```python
from build123d import *

# Parameters (mm, degrees)
PAD002_DEPTH    = 5.1
PAD003_DEPTH    = 5.1
PAD001_DEPTH    = 5.1
SKETCH_W        = 70
SKETCH_H        = 55
PAD_DEPTH       = 10
SKETCH001_R     = 11.05
POCKET_DEPTH    = 7
SKETCH002_R     = 5
POCKET001_DEPTH = 3.001
SKETCH003_W     = 12
SKETCH003_H     = 8.1
SKETCH003_W_2   = 8
SKETCH003_H_2   = 12
POCKET002_DEPTH = 10.001
SKETCH004_R     = 2.1
POCKET003_DEPTH = 10
SKETCH005_R     = 2.1
POCKET004_DEPTH = 10
SKETCH006_R     = 2.1
POCKET005_DEPTH = 10
SKETCH010_W     = 70
SKETCH010_H     = 13
POCKET006_DEPTH = 10.001
SKETCH011_R     = 9
SKETCH011_R_2   = 6
SKETCH011_R_3   = 7
SKETCH011_R_4   = 2.6
PAD004_DEPTH    = 0.3
SKETCH012_R     = 5
PAD005_DEPTH    = 0.3


with BuildPart() as pad002:
    # Sketch008 → Pad002 (new body)
    with BuildSketch(Plane.YZ.offset(24)):
        Polygon((7.570319, 5), (5.53516, 8.525), (1.46484, 8.525), (-0.570319, 5), (-0.570319, 0), (7.570319, 0), align=None)
    extrude(amount=-PAD002_DEPTH)


with BuildPart() as pad003:
    # Sketch009 → Pad003 (new body)
    with BuildSketch(Plane.XZ.offset(16.5)):
        Polygon((-24.929681, 5), (-26.96484, 8.525), (-31.03516, 8.525), (-33.070319, 5), (-33.070319, 0), (-24.929681, 0), align=None)
        Polygon((33.070319, 5), (31.03516, 8.525), (26.96484, 8.525), (24.929681, 5), (24.929681, 0), (33.070319, 0), align=None)
    extrude(amount=-PAD003_DEPTH)


with BuildPart() as pad001:
    # Sketch007 → Pad001 (new body)
    with BuildSketch(Plane.YZ.offset(-24)):
        Polygon((7.570319, 5), (5.53516, 8.525), (1.46484, 8.525), (-0.570319, 5), (-0.570319, 0), (7.570319, 0), align=None)
    extrude(amount=PAD001_DEPTH)


with BuildPart() as obj1:
    # Sketch → Pad (new body)
    with BuildSketch(Plane.XY):
        Rectangle(SKETCH_W, SKETCH_H)
    extrude(amount=PAD_DEPTH)

    # Sketch001 → Pocket (cut)
    with BuildSketch(Plane(origin=(0, 0, 0), x_dir=(1, 0, 0), z_dir=(0, 0, -1))):
        with Locations((0, 13.45)):
            Circle(SKETCH001_R)
    extrude(amount=-POCKET_DEPTH, mode=Mode.SUBTRACT)

    # Sketch002 → Pocket001 (cut, through all)
    with BuildSketch(Plane(origin=(0, 0, 7), x_dir=(1, 0, 0), z_dir=(0, 0, -1))):
        with Locations((0, 13.45)):
            Circle(SKETCH002_R)
    extrude(amount=-POCKET001_DEPTH, mode=Mode.SUBTRACT)

    # Sketch003 → Pocket002 (cut, through all)
    with BuildSketch(Plane.XY.offset(10)):
        with Locations((-29, -23.45)):
            Rectangle(SKETCH003_W, SKETCH003_H)
        with Locations((29, -23.45)):
            Rectangle(SKETCH003_W, SKETCH003_H)
        with Locations((-31, 3.5)):
            Rectangle(SKETCH003_W_2, SKETCH003_H_2)
        with Locations((31, 3.5)):
            Rectangle(SKETCH003_W_2, SKETCH003_H_2)
    extrude(amount=-POCKET002_DEPTH, mode=Mode.SUBTRACT)

    # Sketch004 → Pocket003 (cut)
    with BuildSketch(Plane(origin=(-27, 0, 0), x_dir=(0, -1, 0), z_dir=(-1, 0, 0))):
        with Locations((-3.5, 5)):
            Circle(SKETCH004_R)
    extrude(amount=-POCKET003_DEPTH, mode=Mode.SUBTRACT)

    # Sketch005 → Pocket004 (cut)
    with BuildSketch(Plane.YZ.offset(27)):
        with Locations((3.5, 5)):
            Circle(SKETCH005_R)
    extrude(amount=-POCKET004_DEPTH, mode=Mode.SUBTRACT)

    # Sketch006 → Pocket005 (cut)
    with BuildSketch(Plane.XZ.offset(19.4)):
        with Locations((-29, 5)):
            Circle(SKETCH006_R)
        with Locations((29, 5)):
            Circle(SKETCH006_R)
    extrude(amount=-POCKET005_DEPTH, mode=Mode.SUBTRACT)

    # Cut: cut Pad001
    add(pad001.part, mode=Mode.SUBTRACT)

    # Cut001: cut Pad003
    add(pad003.part, mode=Mode.SUBTRACT)

    # Cut002: cut Pad002
    add(pad002.part, mode=Mode.SUBTRACT)

    # Sketch010 → Pocket006 (cut, through all)
    with BuildSketch(Plane.XY.offset(10)):
        with Locations((0, 21)):
            Rectangle(SKETCH010_W, SKETCH010_H)
    extrude(amount=-POCKET006_DEPTH, mode=Mode.SUBTRACT)

    # Sketch011 → Pad004 (new body)
    with BuildSketch(Plane(origin=(0, 0, 0), x_dir=(1, 0, 0), z_dir=(0, 0, -1))):
        with Locations((-35, -14.5)):
            Circle(SKETCH011_R)
        with Locations((-35, 2.5)):
            Circle(SKETCH011_R_2)
        with Locations((-23, 27.5)):
            Circle(SKETCH011_R_3)
        with Locations((-35, 19.4)):
            Circle(SKETCH011_R_4)
        with Locations((35, 19.4)):
            Circle(SKETCH011_R_4)
        with Locations((23, 27.5)):
            Circle(SKETCH011_R_3)
        with Locations((35, 2.5)):
            Circle(SKETCH011_R_2)
        with Locations((35, -14.5)):
            Circle(SKETCH011_R)
    extrude(amount=-PAD004_DEPTH)

    # Sketch012 → Pad005 (new body)
    with BuildSketch(Plane(origin=(0, 0, 7), x_dir=(1, 0, 0), z_dir=(0, 0, -1))):
        with Locations((0, 13.45)):
            Circle(SKETCH012_R)
    extrude(amount=-PAD005_DEPTH)


solid = obj1.part
```
Can you work these out from the model? Positions are in its coordinate system, mm. A direction names the side the tool comes from. Coordinates: 2 decimals unless noted, no trailing zeros. Loops run counter-clockwise (first coordinate to the right, second up) from the corner with the lowest first, then second, coordinate; pieces in that order, holes last.
1) I need wall thicknesses on probe 1 along Y at (x, z) = (28.5, 2); probe 2 along Y at (x, z) = (18, 5.25); probe 3 along Z at (x, y) = (29, -18.3). Which ranges of each line are inside material? Lowest first, please.
2) Imagine slicing it at B-B on y = -30. List the corners of the cut face in (x, z) for me, plus the area to 3 significant figures.
3) Which directions (+Z, -Z, +X, -X, +Y, -Y) give clear straight access to the entire face, cutting with the end or side of a thin tool? Please do faces 3 (the cylindrical face through (-31.1, -17.97, 5.09)), 4 (the cylindrical face through (-25.521, 3.773, 7.082)), 5 (the flat face through (21, 7.57, 2)), 6 (the cylindrical face through (-0.7, -18.4, 8.6)).
4) Imagine slicing it at A-A on x = 0. List the corners of the cut face in (y, z) for me, plus the area to 3 significant figures.
5) Thinking about a two-plate mould opening in X: for faces 1 (the cylindrical face through (-17.963, 3.773, 7.082)), 2 (the flat face through (-33.07, -14, 3)), which applies, pulls with the +X half, pulls with the -X half, needs draft (parallel to the pull), parting line crosses it, or undercut?
6) Imagine slicing it at D-D on x = 9. List the corners of the cut face in (y, z) for me.
7) For pin 1 (5.5 mm diameter, centred on x = 22.5, z = 3, fed in from +Y); pin 2 (2 mm diameter, centred on x = -28, y = -22, fed in from +Z); pin 3 (1.5 mm diameter, centred on y = -14.5, z = 2, fed in from +X), each with a flat end and sliding along its axis, tell me the tip position at first contact or that it passes through.
8) Imagine slicing it at C-C on y = -7.5. List the corners of the cut face in (x, z) for me.
Completed:
1. probe 1: y = -19.4 to -16.5, -11.4 to -2.5, 9.5 to 14.5
1. probe 2: y = -27.5 to 1.41, 5.59 to 14.5
1. probe 3: z = 0 to 2.9, 7.1 to 10
2. outline: (-29.54, 0) - (-16.46, 0) - (-16.46, 0.3) - (-29.54, 0.3) - close; (16.46, 0) - (29.54, 0) - (29.54, 0.3) - (16.46, 0.3) - close
2. area: 7.85 mm2
3. face 3: -Y
3. face 4: -X
3. face 5: -Z
3. face 6: +Z
4. outline: (-27.5, 0) - (-24.5, 0) - (-24.5, 7) - (-2.4, 7) - (-2.4, 0) - (14.5, 0) - (14.5, 10) - (-8.45, 10) - (-8.45, 7.3) - (-18.45, 7.3) - (-18.45, 10) - (-27.5, 10) - close
4. area: 238 mm2
5. face 1: needs draft
5. face 2: undercut
6. outline: (-27.5, 0) - (-19.86, 0) - (-19.86, 7) - (-7.04, 7) - (-7.04, 0) - (14.5, 0) - (14.5, 10) - (-27.5, 10) - close
7. pin 1: stops at y = 14.5
7. pin 2: stops at z = 0.3
7. pin 3: stops at x = 35
8. outline: (-38.32, 0) - (-9.31, 0) - (-9.31, 7) - (9.31, 7) - (9.31, 0) - (38.32, 0) - (38.32, 0.3) - (35, 0.3) - (35, 10) - (-35, 10) - (-35, 0.3) - (-38.32, 0.3) - close
